```python
from build123d import *

# Parameters (mm, degrees)
SKETCH1_R           = 1
BOSS_EXTRUDE1_DEPTH = 2
BOSS_EXTRUDE2_START = 8
BOSS_EXTRUDE2_DEPTH = 6.8
SKETCH3_W           = 2.8
SKETCH3_H           = 2
SKETCH3_W_2         = 5.8
BOSS_EXTRUDE3_DEPTH = 11


with BuildPart() as part:
    # Sketch1 → Boss-Extrude1 (new body)
    with BuildSketch(Plane(origin=(0, 0, 0), x_dir=(1, 0, 0), z_dir=(0, 1, 0))):
        with BuildLine():
            Line((11.7, 3), (11.7, 7.6))
            ThreePointArc((11.7, 7.6), (11.407106781, 8.307106781), (10.7, 8.6))
            Line((10.7, 8.6), (-10.3, 8.6))
            ThreePointArc((-10.3, 8.6), (-11.007106781, 8.307106781), (-11.3, 7.6))
            Line((-11.3, 7.6), (-11.3, -8))
            Line((-11.3, -8), (-6.6, -8))
            Line((-6.6, -8), (-6.6, 0))
            Line((-6.6, 0), (6.6, 0))
            ThreePointArc((6.6, 0), (7.478679656, 2.121320344), (9.6, 3))
            Line((9.6, 3), (11.7, 3))
        make_face()
        with Locations((8.7, 5.469565217)):
            Circle(SKETCH1_R, mode=Mode.SUBTRACT)
        with Locations((-8.3, 5.469565217)):
            Circle(SKETCH1_R, mode=Mode.SUBTRACT)
    extrude(amount=BOSS_EXTRUDE1_DEPTH)

    # Sketch2 → Boss-Extrude2 (add)
    with BuildSketch(Plane.XY.offset(BOSS_EXTRUDE2_START)):
        Polygon((-9, 2), (-9, 12.1), (-10.5, 12.1), (-10.5, 14.1), (-4.7, 14.1), (-4.7, 12.1), (-6.2, 12.1), (-6.2, 2), align=None)
    extrude(amount=-BOSS_EXTRUDE2_DEPTH)

    # Sketch3 → Boss-Extrude3 (add)
    with BuildSketch(Plane.XY.offset(8)):
        with Locations((-7.6, 13.1)):
            Rectangle(SKETCH3_W, SKETCH3_H)
        with Locations((-7.6, 6.9)):
            Rectangle(SKETCH3_W_2, SKETCH3_H)
    extrude(amount=-BOSS_EXTRUDE3_DEPTH)


solid = part.part
```
Geometry check sheet. Reference: the model listing, model coordinates, mm. A direction names the side the tool comes from. Coordinates: 2 decimals unless noted, no trailing zeros. Write each loop counter-clockwise with the first axis right and the second up, starting at its lowest first coordinate (ties: lowest second). Pieces come first, ordered by that corner, then holes. Notation, with made-up numbers: (-16, 29.25) -> (39, 29.25) arc R20 ccw to (39, 48.25) -> close; hole circle Ø4 at (-19, 37). An arc over 180 degrees is marked (long way). Use CSV: the item, a comma, the result in double quotes. Start each with the question number.
Item 1: Cross-section at B-B, the plane x = -5.25. Record the cut outline in (y, z).
Item 2: Cross-section at A-A, the plane x = -8.3. Record the cut outline in (y, z).
Item 3: Depth check by flat-ended pin: pin 1 Ø1.6 at (x, y) = (10.5, 1) entering from +Z; pin 2 Ø1.7 at (x, z) = (-6.5, 4) entering from -Y; pin 3 Ø3 at (x, y) = (-8, 10.5) entering from -Z; pin 4 Ø6 at (x, z) = (9, 0.5) entering from +Y. Enter the tip coordinate at first touch or a pass-through.
Item 4: Set-up check for faces 5 (the flat face through (-8, 4, 1.2)), 6 (the flat face through (-6.6, 1, 4)), 7 (the flat face through (-8, 13, -3)), 8 (the flat face through (-5, 12.1, 5)): record each of +Z, -Z, +X, -X, +Y, -Y from which the full face is reachable in a straight line by a thin tool's end or side.
Item 5: Thickness scan on line 1 (Y direction, x = -9.5, z = 6.75); line 2 (Y direction, x = -6, z = -2.5); line 3 (Z direction, x = -8.3, y = 1.2). Record the ranges inside material, lowest first.
Item 6: Mould release check, pull along Y, two halves, no side actions. Record for faces 1 (the flat face through (-8, 14.1, 4)), 2 (the flat face through (-8, 7.9, 0)), 3 (the flat face through (-3, 2, -4)), 4 (the cylindrical face through (-10.999, 0.986, -8.315)): released by +Y, released by -Y, zero draft, split by the parting line, or undercut.
Item 7: Cross-section at D-D, the plane z = 1.5. Record the cut outline in (x, y).
Item 8: Cross-section at C-C, the plane z = -6. Record the cut outline in (x, y), plus the area to 3 significant figures.
Answers:
1,outline,"(0, -8.6) -> (2, -8.6) -> (2, 0) -> (0, 0) -> close; (5.9, -3) -> (7.9, -3) -> (7.9, 8) -> (5.9, 8) -> close; (12.1, 1.2) -> (14.1, 1.2) -> (14.1, 8) -> (12.1, 8) -> close"
2,outline,"(0, -8.6) -> (2, -8.6) -> (2, -6.47) -> (0, -6.47) -> close; (0, -4.47) -> (2, -4.47) -> (2, 1.2) -> (5.9, 1.2) -> (5.9, -3) -> (7.9, -3) -> (7.9, 1.2) -> (12.1, 1.2) -> (12.1, -3) -> (14.1, -3) -> (14.1, 8) -> (0, 8) -> close"
3,pin 1,"z = -3"
3,pin 2,"y = 0"
3,pin 3,"z = 1.2"
3,pin 4,"y = 2"
4,face 5,"-Z, +X, -X"
4,face 6,"+Z, +X, -Y"
4,face 7,"-Z, +X, -X, +Y"
4,face 8,"+Z, -Z, +X"
5,line 1,"0 to 2, 5.9 to 7.9, 12.1 to 14.1"
5,line 2,"0 to 2, 5.9 to 7.9"
5,line 3,"-8.6 to -6.47, -4.47 to 8"
6,face 1,"released by +Y"
6,face 2,"undercut"
6,face 3,"undercut"
6,face 4,"zero draft"
7,outline,"(-11.3, 0) -> (-6.6, 0) -> (-6.6, 2) -> (-6.2, 2) -> (-6.2, 5.9) -> (-4.7, 5.9) -> (-4.7, 7.9) -> (-6.2, 7.9) -> (-6.2, 12.1) -> (-4.7, 12.1) -> (-4.7, 14.1) -> (-10.5, 14.1) -> (-10.5, 12.1) -> (-9, 12.1) -> (-9, 7.9) -> (-10.5, 7.9) -> (-10.5, 5.9) -> (-9, 5.9) -> (-9, 2) -> (-11.3, 2) -> close"
8,outline,"(-11.3, 0) -> (-9.15, 0) -> (-9.15, 2) -> (-11.3, 2) -> close; (-7.45, 0) -> (7.85, 0) -> (7.85, 2) -> (-7.45, 2) -> close; (9.55, 0) -> (11.7, 0) -> (11.7, 2) -> (9.55, 2) -> close"
8,area,"39.2 mm^2"
